Autodesk Inventor part; units mm, degrees
ref_plane "YZ Plane" through (0, 0, 0) normal (1, 0, 0) x (0, 1, 0)
ref_plane "XZ Plane" through (0, 0, 0) normal (0, 1, 0) x (-1, 0, 0)
ref_plane "XY Plane" through (0, 0, 0) normal (0, 0, 1) x (1, 0, 0)
sketch "Sketch1" plane through (0, 0, 0) normal (0, 1, 0) x (-1, 0, 0)
  line L0 (40, 20) -> (80, 20)
  line L1 (80, 20) -> (80, -20)
  line L2 (80, -20) -> (40, -20)
  line L3 (40, -20) -> (40, 20)
  circle A0 centre (60, 0) radius 2.75
  line L4 (40, -86) -> (-165.5, -86)
  line L5 (-165.5, -86) -> (-165.5, 86)
  line L6 (-165.5, 86) -> (40, 86)
  line L7 (40, 86) -> (40, -86)
  line L8 (-165.5, -86) -> (-90.5, -86)
  line L9 (-90.5, -86) -> (-90.5, -71)
  line L10 (-90.5, -71) -> (-165.5, -71)
  line L11 (-165.5, -71) -> (-165.5, -86)
  line L12 (-165.5, 86) -> (-90.5, 86)
  line L13 (-90.5, 86) -> (-90.5, 71)
  line L14 (-90.5, 71) -> (-165.5, 71)
  line L15 (-165.5, 71) -> (-165.5, 86)
  circle A1 centre (-27.75, 0) radius 2.75
  circle A2 centre (-27.75, 45.5) radius 2.75
  circle A3 centre (-27.75, -45.5) radius 2.75
  circle A4 centre (-115.5, 0) radius 2.75
  point P0 (-165.5, 0)
  dimension "d0" = 40
  dimension "d1" = 40
  dimension "d7" = 5.5
  dimension "d24" = 75
  dimension "d25" = 15
  dimension "d26" = 75
  dimension "d27" = 15
  dimension "d29" = 5.5
  dimension "d30" = 5.5
  dimension "d31" = 5.5
  dimension "d32" = 5.5
extrude "Extrusion1" add sketch "Sketch1" along normal blind 3 contours L0 L1 L2 L3 | L3 L7 L4 L9 L10 L5 L14 L13 L6
fillet "Fillet6" radius 20 6 edges at (90.5, 1.5, 86) (90.5, 1.5, 71) (165.5, 1.5, 71) (90.5, 1.5, -86) (90.5, 1.5, -71) (165.5, 1.5, -71)
properties part number "Chassis Front Plate"
Could you check a few things on this model? Use its own coordinates, in mm. Round coordinates to 2 decimals unless told otherwise and drop trailing zeros. Loops run counter-clockwise (first coordinate to the right, second up) from the corner with the lowest first, then second, coordinate; pieces in that order, holes last.
Q1. Please list where these lines run through material, in increasing order: L1, parallel to Z at x = 27.75, y = 1.4; L2, parallel to Z at x = 115.5, y = 2.3; L3, parallel to Z at x = -48.5, y = 2.5.
Q2. I want a section at D-D (z = 0). Write out the boundary of the cut face in (x, y).
Q3. I want a section at B-B (x = -60). Write out the boundary of the cut face in (y, z).
Q4. I want a section at A-A (z = -45.5). Write out the boundary of the cut face in (x, y), and give its area (3 significant figures).
Q5. Thinking about a two-plate mould opening in X: for faces 1 (the cylindrical face through (159.486, 1.479, -65.297)), 2 (the cylindrical face through (118.247, 1.479, -0.121)), 3 (the flat face through (44, 0, 1)), which applies, pulls with the +X half, pulls with the -X half, needs draft (parallel to the pull), parting line crosses it, or undercut?
Q6. For P1, Ø0.9, axis at x = 132, y = 2, coming from the -Z side; P2, Ø0.9, axis at x = -50, y = 1.5, coming from the +Z side; P3, Ø3.5, axis at x = 27.75, z = 0, coming from the +Y side, each with a flat end and sliding along its axis, tell me the tip position at first contact or that it passes through.
Q7. I want a section at C-C (y = 2.15). Write out the boundary of the cut face in (x, z), and give its area (3 significant figures).
Answer below:
1. L1: z = -86 to -48.25, -42.75 to -2.75, 2.75 to 42.75, 48.25 to 86
1. L2: z = -71 to -2.75, 2.75 to 71
1. L3: z = -20 to 20
2. outline: (-80, 0) - (-62.75, 0) - (-62.75, 3) - (-80, 3) - close; (-57.25, 0) - (25, 0) - (25, 3) - (-57.25, 3) - close; (30.5, 0) - (112.75, 0) - (112.75, 3) - (30.5, 3) - close; (118.25, 0) - (165.5, 0) - (165.5, 3) - (118.25, 3) - close
3. outline: (0, -20) - (3, -20) - (3, -2.75) - (0, -2.75) - close; (0, 2.75) - (3, 2.75) - (3, 20) - (0, 20) - close
4. outline: (-40, 0) - (25, 0) - (25, 3) - (-40, 3) - close; (30.5, 0) - (165.5, 0) - (165.5, 3) - (30.5, 3) - close
4. area: 600 mm2
5. face 1: pulls with the +X half
5. face 2: undercut
5. face 3: needs draft
6. P1: stops at z = -71
6. P2: stops at z = 20
6. P3: passes through
7. outline: (-80, -20) - (-40, -20) - (-40, -86) - (78.64, -86) arc R20 ccw to (94.25, -78.5) arc R20 cw to (109.86, -71) - (145.5, -71) arc R20 ccw to (165.5, -51) - (165.5, 51) arc R20 ccw to (145.5, 71) - (109.86, 71) arc R20 cw to (94.25, 78.5) arc R20 ccw to (78.64, 86) - (-40, 86) - (-40, 20) - (-80, 20) - close; hole circle Ø5.5 at (-60, 0); hole circle Ø5.5 at (27.75, -45.5); hole circle Ø5.5 at (27.75, 0); hole circle Ø5.5 at (27.75, 45.5); hole circle Ø5.5 at (115.5, 0)
7. area: 34,500 mm2
